CAD build for the part. Positions are in the model's coordinates, mm. A direction names the side the tool comes from. Coordinates: 2 decimals unless noted, no trailing zeros. Order: outer loops, then holes, each group sorted by start corner. A loop starts at its lowest first (then second) coordinate and runs counter-clockwise, first axis right, second up. Notation, with made-up numbers: (82, -14.75) - (123, -14.75) arc R18 ccw to (123, 2.25) - close; hole circle Ø2 at (85, 51). An arc over 180 degrees is marked (long way). Use one line per item in the form item = value.
Autodesk Inventor part; units mm, degrees
ref_plane "YZ Plane" through (0, 0, 0) normal (1, 0, 0) x (0, 1, 0)
ref_plane "XZ Plane" through (0, 0, 0) normal (0, 1, 0) x (-1, 0, 0)
ref_plane "XY Plane" through (0, 0, 0) normal (0, 0, 1) x (1, 0, 0)
sketch "Sketch1" plane through (0, 0, 0) normal (0, 0, 1) x (1, 0, 0)
  line L0 (0, 0) -> (0, 2.413)
  line L1 (0, 2.413) -> (-4.826, 2.413)
  line L2 (-4.826, 2.413) -> (-4.826, 3.175)
  line L3 (-4.826, 3.175) -> (-11.176, 3.175)
  line L4 (-11.176, 3.175) -> (-11.176, 3.81)
  line L5 (-11.176, 3.81) -> (-9.906, 3.81)
  line L6 (-9.906, 3.81) -> (-9.906, 3.556)
  line L7 (-9.906, 3.556) -> (0.254, 3.6741)
  line L8 (0.254, 3.6741) -> (0.254, 5.842)
  line L9 (0.254, 5.842) -> (-4.064, 5.842)
  line L10 (-4.064, 5.842) -> (-4.064, 7.239)
  line L11 (-4.064, 7.239) -> (1.016, 7.239)
  line L12 (1.016, 7.239) -> (1.016, 3.683)
  line L13 (1.016, 3.683) -> (3.556, 3.683)
  line L14 (3.556, 3.683) -> (3.556, 3.81)
  line L15 (3.556, 3.81) -> (5.08, 3.683)
  line L16 (5.08, 3.683) -> (5.08, 3.81)
  line L17 (5.08, 3.81) -> (6.604, 3.683)
  line L18 (6.604, 3.683) -> (6.604, 3.81)
  line L19 (6.604, 3.81) -> (8.128, 3.683)
  line L20 (8.128, 3.683) -> (10.668, 3.683)
  line L21 (10.668, 3.683) -> (10.668, 3.175)
  line L22 (10.668, 3.175) -> (9.398, 3.175)
  line L23 (9.398, 3.175) -> (9.398, 2.413)
  line L24 (9.398, 2.413) -> (1.057, 2.413)
  line L25 (1.057, 2.413) -> (1.057, 0)
  line L26 (1.057, 0) -> (0, 0)
  dimension "d0" = 21.844
  dimension "d1" = 1.27
  dimension "d2" = 6.35
  dimension "d3" = 11.43
  dimension "d4" = 5.08
  dimension "d5" = 1.524
  dimension "d6" = 1.524
  dimension "d7" = 1.524
  dimension "d8" = 1.27
  dimension "d9" = 2.54
  dimension "d10" = 2.54
  dimension "d11" = 4.826
  dimension "d13" = 5.842
  dimension "d14" = 7.239
  dimension "d15" = 0.254
  dimension "d16" = 0.127
  dimension "d17" = 0.127
  dimension "d18" = 2.413
  dimension "d19" = 3.175
  dimension "d20" = 3.683
  dimension "d21" = 3.81
  dimension "d22" = 3.175
  dimension "d23" = 2.413
revolve "Revolution1" add sketch "Sketch1" angle 360 about axis through (1.057, 0, 0) along (-1, 0, 0)
sketch "Sketch2" plane through (-11.176, 0, 0) normal (-1, 0, 0) x (0, 0, 1)
  circle A0 centre (0, 0) radius 3.81
  line L0 (0.4164, -4.7623) -> (-0.5996, -4.7623)
  line L1 (-0.5996, -4.7623) -> (-0.5996, 4.4311)
  line L2 (-0.5996, 4.4311) -> (0.4164, 4.4311)
  line L3 (0.4164, 4.4311) -> (0.4164, -4.7623)
  dimension "d25" = 1.016
extrude "Extrusion1" cut sketch "Sketch2" against normal blind 5.08 contours L3 A0 L1 | A0 L1 L2 L3 | L3 L0 L1 A0
equation "\"d6\" = d5"
equation "\"d7\" = d6"
properties part number "ARTHURW5.5a AXLE"
Item 1: Drill centre lines: line 1 (Z direction, x = -1.35, y = 0); line 2 (Y direction, x = -1.5, z = -0.25); line 3 (Z direction, x = -6.25, y = 0) (1 decimal). Where is each one in solid material? Low to high. Write a range as [from, to].
Derived:
line_1 = [-7.24, -5.84], [-3.66, -2.41], [2.41, 3.66], [5.84, 7.24]
line_2 = [-7.23, -5.84], [-3.65, -2.4], [2.4, 3.65], [5.84, 7.23]
line_3 = [-3.6, -3.2], [3.2, 3.6]
Item 2: Drop flat-ended pins along their axis: pin 1 (5.5 mm diameter, centred on y = 0, z = -1, fed in from +X); pin 2 (4 mm diameter, centred on y = 0, z = 0, fed in from -X); pin 3 (1 mm diameter, centred on y = 0.5, z = 2, fed in from +X); pin 4 (3 mm diameter, centred on x = 2, y = -2, fed in from +Z). Give the stop position or say it passes through.
Derived:
pin_1 = 10.67
pin_2 = 0
pin_3 = 9.4
pin_4 = 7.19
Item 3: Two-plate mould, pull along Z, no slides. Class faces 4 (the face through (-11.176, -0.3, 3.4)), 5 (the face through (6.17, -2.741, -2.514)), 6 (the face through (1.057, 0, 0)): +Z half, -Z half, draft (parallel to the pull), parting line (faces both ways), or undercut.
Derived:
face_4 = draft
face_5 = parting line
face_6 = undercut
Item 4: 3-axis set-ups, long thin cutter, end or side, ignore diameter. For faces 1 (the face through (4.646, -2.741, -2.514)), 2 (the face through (10.02, -0.69, 3.1)), 3 (the face through (-8.05, 3.03, -0.95)): which of +Z, -Z, +X, -X, +Y, -Y reach the whole face in a straight line?
Derived:
face_1 = none
face_2 = +X
face_3 = -X
Item 5: Cut at A-A, the plane x = -7. Write the cut outline in (y, z) (3 decimals).
Derived:
outline = (-3.566, 0.416) - (-3.148, 0.416) arc R3.175 cw to (3.148, 0.416) - (3.566, 0.416) arc R3.59 ccw to start; (-3.539, -0.6) arc R3.59 ccw to (3.539, -0.6) - (3.118, -0.6) arc R3.175 cw to (-3.118, -0.6) - close
Item 6: Cut at D-D, the plane x = 1.5. Write the cut outline in (y, z), plus the area to 3 significant figures.
Derived:
outline = circle Ø7.37 at (0, 0); hole circle Ø4.83 at (0, 0)
area = 24.3 mm²
Item 7: Cut at B-B, the plane y = 4.25. Write the cut outline in (x, z).
Derived:
outline = (-4.06, -5.86) - (1.02, -5.86) - (1.02, 5.86) - (-4.06, 5.86) - (-4.06, 4.01) - (0.25, 4.01) - (0.25, -4.01) - (-4.06, -4.01) - close
